The listing builds one solid part. Answer for the finished solid, in the listing's coordinates (mm). Round coordinates to 2 decimals unless told otherwise and drop trailing zeros. Order: outer loops, then holes, each group sorted by start corner. A loop starts at its lowest first (then second) coordinate and runs counter-clockwise, first axis right, second up. Notation, with made-up numbers: (-39.75, 44) - (-12.75, 44) arc R5 cw to (-12.75, 53) - close; hole circle Ø9 at (-2.5, -15.5). An arc over 180 degrees is marked (long way). Write item = value, one per line.
Autodesk Inventor part; units mm, degrees
ref_plane "YZ Plane" through (0, 0, 0) normal (1, 0, 0) x (0, 1, 0)
ref_plane "XZ Plane" through (0, 0, 0) normal (0, 1, 0) x (-1, 0, 0)
ref_plane "XY Plane" through (0, 0, 0) normal (0, 0, 1) x (1, 0, 0)
sketch "Sketch1" plane through (0, 0, 0) normal (0, 0, 1) x (1, 0, 0)
  circle A0 centre (0, 0) radius 100
  dimension "d22" = 200
extrude "Plate1" add sketch "Sketch1" along normal blind 3
sketch "Sketch5" plane through (0, 0, 3) normal (0, 0, 1) x (1, 0, 0)
  circle A0 centre (0, 0) radius 100
  circle A1 centre (0, 80) radius 9
  dimension "d23" = 18
  dimension "d24" = 80
extrude "Cut1" cut sketch "Sketch5" against normal blind 3 contours A1
pattern_circular "Circular Pattern1" count 8 over 360 about axis through (0, 0, 0) along (0, 0, 1) of "Cut1"
equation "\"d25\" = Thickness"
equation "\"d2\" = Thickness"
equation "\"BendReliefWidth\" = Thickness"
equation "\"BendReliefDepth\" = 0.5 * Thickness"
equation "\"CornerReliefSize\" = 4 * Thickness"
equation "\"MinimumRemnant\" = 2 * Thickness"
equation "\"TransitionRadius\" = BendRadius"
equation "\"JacobiRadiusSize\" = BendRadius"
equation "\"GapSize\" = Thickness"
properties part number "MSC 920 plug 88.9" material "Stainless Steel"
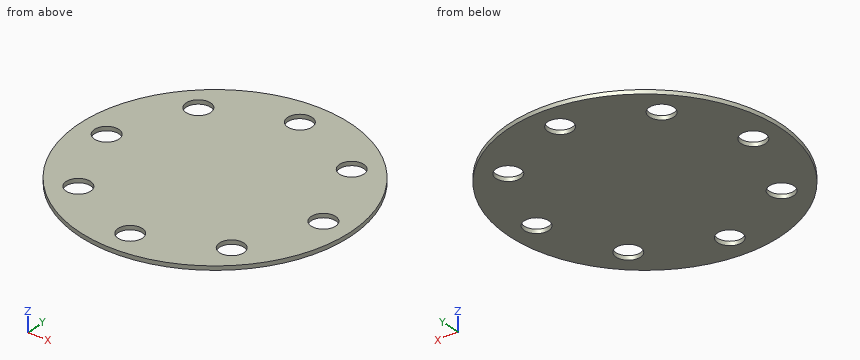
Q1. Section B-B on x = 0 is taken. Determine the outline of the cut face in (y, z), then the cut area to 3 significant figures.
Model answer:
outline = (-100, 0) - (-89, 0) - (-89, 3) - (-100, 3) - close; (-71, 0) - (71, 0) - (71, 3) - (-71, 3) - close; (89, 0) - (100, 0) - (100, 3) - (89, 3) - close
area = 492 mm^2
Q2. Section A-A on y = -80 is taken. Determine the outline of the cut face in (x, z), then the cut area to 3 significant figures.
Model answer:
outline = (-60, 0) - (-9, 0) - (-9, 3) - (-60, 3) - close; (9, 0) - (60, 0) - (60, 3) - (9, 3) - close
area = 306 mm^2
Q3. Flat-ended cylindrical pins translate along their axes: P1, Ø1.5, axis at y = 7.5, z = 2, coming from the +X side; P2, Ø1.5, axis at x = -75, z = 2, coming from the +Y side. Find the tip coordinate at first contact, or state that the pin passes through.
Model answer:
P1 = 99.77
P2 = 66.98
Q4. Find the intervals of material crossed by line 1 (Y direction, x = 0, z = 1.55); line 2 (Y direction, x = -7, z = 0.7); line 3 (X direction, y = 61, z = 0.3), in increasing order. Write a range as from..to.
Model answer:
line_1 = -100..-89, -71..71, 89..100
line_2 = -99.75..-85.66, -74.34..74.34, 85.66..99.75
line_3 = -79.24..-64.4, -48.74..48.74, 64.4..79.24
